For this review, take the finished solid that the model builds, in its own axes (mm). Face numbers are marked on the shaded views. Round coordinates to 2 decimals unless told otherwise and drop trailing zeros.
1) Mouldability with a two-part tool opening along Z and no side actions: class the marked faces 1 and 2 as pulls with the +Z half, pulls with the -Z half, needs draft (parallel to the pull), parting line crosses it, or undercut.
2) Insertion check: pin 1 (2 mm diameter, centred on x = 274, z = -1, fed in from -Y). The pin has a flat end and moves straight along its axis. Give the tip position at first contact, or say it passes through.
3) Take a section at A-A (z = -2.6). Give the number of separate pieces and of enclosed holes in the cut face, then the cut area to 3 significant figures.
4) Wall thickness on L1, parallel to Y at x = 273, z = -1.15; L2, parallel to Y at x = 521, z = -1.45; L3, parallel to X at y = 38, z = -2.8: over which ranges is each line inside the solid? List them lowest first.
```python
from build123d import *

# Parameters (mm, degrees)
SCHIZZO1_W                   = 526
SCHIZZO1_H                   = 75
SCHIZZO1_R                   = 2
ESTRUSIONE_ESTRUSIONE1_DEPTH = 4
SCHIZZO2_R                   = 2
TAGLIO_ESTRUSIONE1_DEPTH     = 4


with BuildPart() as part:
    # Schizzo1 → Estrusione-Estrusione1 (new body)
    with BuildSketch(Plane.XY):
        with Locations((263, 37.5)):
            Rectangle(SCHIZZO1_W, SCHIZZO1_H)
        with Locations((5, 37.5)):
            Circle(SCHIZZO1_R, mode=Mode.SUBTRACT)
        with Locations((5, 65)):
            Circle(SCHIZZO1_R, mode=Mode.SUBTRACT)
        with Locations(Location((5, 10, 0), (0, 0, 180))):
            Circle(SCHIZZO1_R, mode=Mode.SUBTRACT)
        with Locations((521, 10)):
            Circle(SCHIZZO1_R, mode=Mode.SUBTRACT)
        with Locations(Location((521, 65, 0), (0, 0, 180))):
            Circle(SCHIZZO1_R, mode=Mode.SUBTRACT)
        with Locations(Location((521, 37.5, 0), (0, 0, 180))):
            Circle(SCHIZZO1_R, mode=Mode.SUBTRACT)
    extrude(amount=-ESTRUSIONE_ESTRUSIONE1_DEPTH)

    # Schizzo2 → Taglio-Estrusione1 (cut)
    with BuildSketch(Plane.XY):
        with Locations((253, 62.5)):
            Circle(SCHIZZO2_R)
        with Locations(Location((273, 62.5, 0), (0, 0, 180))):
            Circle(SCHIZZO2_R)
        with Locations((253, 42.5)):
            Circle(SCHIZZO2_R)
        with Locations((273, 42.5)):
            Circle(SCHIZZO2_R)
        with BuildLine():
            Line((293, -15), (293, 11))
            ThreePointArc((293, 11), (291.828427125, 13.828427125), (289, 15))
            Line((289, 15), (237, 15))
            ThreePointArc((237, 15), (234.171572875, 13.828427125), (233, 11))
            Line((233, 11), (233, -15))
            Line((233, -15), (293, -15))
        make_face()
    extrude(amount=-TAGLIO_ESTRUSIONE1_DEPTH, mode=Mode.SUBTRACT)


solid = part.part
```
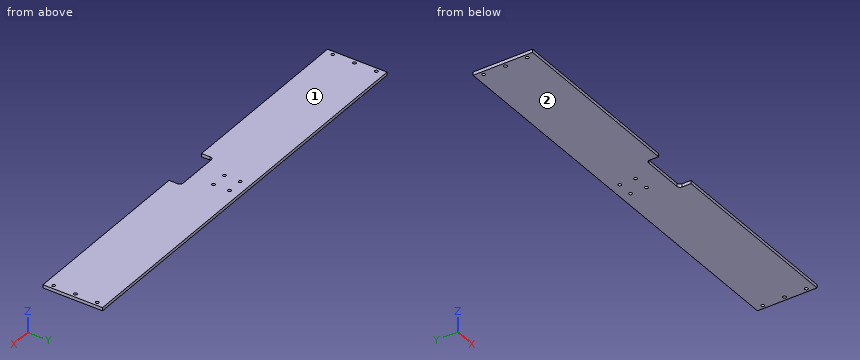
Response:
1. face 1: pulls with the +Z half
1. face 2: pulls with the -Z half
2. pin 1: stops at y = 15
3. separate pieces: 1
3. enclosed holes: 10
3. area: 38,400 mm2
4. L1: y = 15 to 40.5, 44.5 to 60.5, 64.5 to 75
4. L2: y = 0 to 8, 12 to 35.5, 39.5 to 63, 67 to 75
4. L3: x = 0 to 3.06, 6.94 to 519.06, 522.94 to 526
